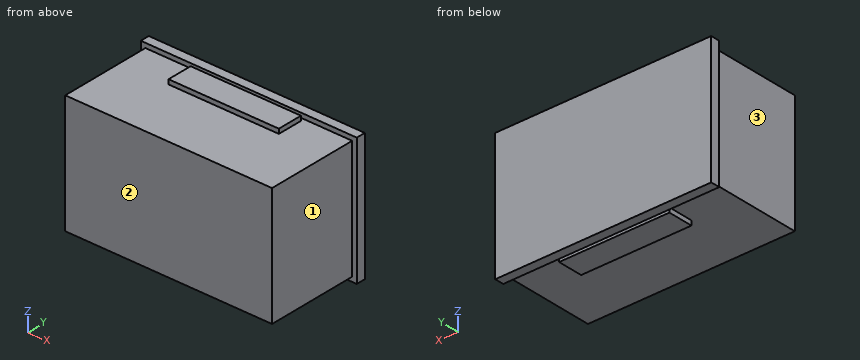
```python
from build123d import *

# Parameters (mm, degrees)
F0_W     = 45
F0_H     = 26
F1_DEPTH = 22
F0_W_2   = 47
F0_H_2   = 28
F2_DEPTH = 2
F3_W     = 24
F3_H     = 5.5
F4_DEPTH = 1


# Not quite as in the source:
# - a pattern or mirror of a feature is missing from the dataset's text; its kind, count and spacing are read off the source's solid


with BuildPart() as f1:
    # F0 (on Front) → F1 (new body)
    with BuildSketch(Plane.XZ):
        Rectangle(F0_W, F0_H)
    extrude(amount=F1_DEPTH)

    # F0 (on Front) → F2 (join)
    with BuildSketch(Plane.XZ):
        Rectangle(F0_W_2, F0_H_2)
        Rectangle(F0_W, F0_H, mode=Mode.SUBTRACT)
    extrude(amount=F2_DEPTH)

    # F3 (on face) → F4 (join)
    with BuildSketch(Plane.XY.offset(13)):
        with Locations((0, -5.5)):
            Rectangle(F3_W, F3_H)
    f4 = extrude(amount=F4_DEPTH)

    # F4_copies: F4 across plane
    add(f4.mirror(Plane(origin=(0, 0, 0), x_dir=(-1, 0, 0), z_dir=(0, 0, -1))))


solid = f1.part
```
Can you work these out from the model? Positions are in its coordinate system, mm. Face numbers are marked on the shaded views. A direction names the side the tool comes from. Round coordinates to 2 decimals unless told otherwise and drop trailing zeros. Order: outer loops, then holes, each group sorted by start corner. A loop starts at its lowest first (then second) coordinate and runs counter-clockwise, first axis right, second up.
(1) If we section it at A-A (y = -4.5): Please give me the cut outline in (x, z), plus the area to 3 significant figures.
Results are:
outline: (-22.5, -13) - (-12, -13) - (-12, -14) - (12, -14) - (12, -13) - (22.5, -13) - (22.5, 13) - (12, 13) - (12, 14) - (-12, 14) - (-12, 13) - (-22.5, 13) - close
area: 1,220 mm2
(2) On a 3-axis mill with a long thin cutter (end or side, diameter ignored), from which of +Z, -Z, +X, -X, +Y, -Y can I reach the whole of each face in a straight line? I mean the marked faces 1, 2 and 3. Say none if no direction works.
Results are:
face 1: +Z, -Z, +X, -Y
face 2: +Z, -Z, +X, -X, -Y
face 3: +Z, -Z, -X, -Y
(3) If I drill on L1, parallel to X at y = -10.5, z = 3.75; L2, parallel to Z at x = 7, y = -17.5, over which ranges is the centre line in solid material (lowest first)?
Results are:
L1: x = -22.5 to 22.5
L2: z = -13 to 13
(4) If we section it at C-C (z = -6.25): Please give me the cut outline in (x, y).
Results are:
outline: (-23.5, -2) - (-22.5, -2) - (-22.5, -22) - (22.5, -22) - (22.5, -2) - (23.5, -2) - (23.5, 0) - (-23.5, 0) - close
(5) I'm going to push flat-ended pins straight in: pin 1 (1 mm diameter, centred on x = 2, y = -17, fed in from +Z); pin 2 (8 mm diameter, centred on x = 12, y = -19, fed in from -Z); pin 3 (6 mm diameter, centred on y = -17, z = 4, fed in from +X). Where does each tip first touch, or does it pass through?
Results are:
pin 1: stops at z = 13
pin 2: stops at z = -13
pin 3: stops at x = 22.5
(6) If we section it at B-B (x = 20): Please give me the cut outline in (y, z), plus the area to 3 significant figures.
Results are:
outline: (-22, -13) - (-2, -13) - (-2, -14) - (0, -14) - (0, 14) - (-2, 14) - (-2, 13) - (-22, 13) - close
area: 576 mm2
(7) If we section it at D-D (x = -3.5): Please give me the cut outline in (y, z).
Results are:
outline: (-22, -13) - (-8.25, -13) - (-8.25, -14) - (-2.75, -14) - (-2.75, -13) - (-2, -13) - (-2, -14) - (0, -14) - (0, 14) - (-2, 14) - (-2, 13) - (-2.75, 13) - (-2.75, 14) - (-8.25, 14) - (-8.25, 13) - (-22, 13) - close
